Input: part model. Units: mm. Frame: model coordinates. A direction names the side the tool comes from. Round coordinates to 2 decimals unless told otherwise and drop trailing zeros. Loops run counter-clockwise (first coordinate to the right, second up) from the corner with the lowest first, then second, coordinate; pieces in that order, holes last. Notation, with made-up numbers: M 27.5,79 L 36.5,79 A25 cw 36.5,102 Z; hole C 47,-7.5 d6. An arc over 180 degrees is marked long. Return JSON: item names as keys, results as strings. Group by question number.
1) Section A-A (x = 47). Output: boundary loops of the cut face in (y, z).
2) Access query for faces 1 (the face through (67.71, -12.64, 2.81)), 2 (the face through (0, 0, 0)), 3 (the face through (137.62, -2.38, 10.74)), 4 (the face through (67, 12, 0)). Directions: +Z, -Z, +X, -X, +Y, -Y. A direction counts if a zero-diameter tool reaches every point of the face in a straight line with its end or side. Return the directions, or none.
3) Contact query for flat-ended pins moving along their axis: P1, Ø6, axis at x = 120.5, z = 9.5, coming from the +Y side; P2, Ø6, axis at y = -14, z = 11.5, coming from the -X side; P3, Ø8, axis at x = 48.5, z = -10, coming from the -Y side. Output: stop coordinate, or through.
4) Section B-B (z = -15.5). Output: boundary loops of the cut face in (x, y).
5) Mould query, pull axis Z, two halves, no side actions, for faces 5 (the face through (42, 12, 4)), 6 (the face through (90, 5, 10)), 7 (the face through (16.014, 8.767, 16.856)). Classes: +Z half, -Z half, draft (parallel to the pull), parting line (faces both ways), or undercut.
6) Material intervals for line 1 (X direction, y = 1.5, z = 13); line 2 (X direction, y = 13.5, z = 1.5); line 3 (X direction, y = 15, z = 2.5), sorted ascending. Write a range as from..to.
from build123d import *

# Parameters (mm, degrees)
CUT_EXTRUDE_START   = 10
CUT_EXTRUDE_1_DEPTH = 132.573302568
CUT_EXTRUDE_START_2 = 7
CUT_EXTRUDE_2_DEPTH = 135.573302568
CUT_EXTRUDE_START_3 = 68.5
SKETCH_4_R          = 14
SKETCH_4_R_2        = 12.95
CUT_EXTRUDE_3_DEPTH = 1.6
CUT_EXTRUDE_START_4 = 136.2
SKETCH_5_R          = 11
SKETCH_5_R_2        = 10.25
CUT_EXTRUDE_4_DEPTH = 1.3


with BuildPart() as part:
    # Эскиз1 → Повернуть1 (revolve)
    with BuildSketch(Plane.XY):
        Polygon((0, 0), (0, 12.5), (15, 12.5), (15, 14), (15, 19), (17, 19), (17, 14), (75, 14), (75, 12.5), (90, 12.5), (90, 11), (139, 11), (139, 0), align=None)
    revolve(axis=Axis((139, 0, 0), (-1, 0, 0)))

    # Эскиз2 → Вырез-Вытянуть1 (cut, through all)
    with BuildSketch(Plane(origin=(0, 0, 0), x_dir=(1, 0, 0), z_dir=(0, 1, 0)).offset(CUT_EXTRUDE_START)):
        with BuildLine():
            Line((21, 4), (63, 4))
            ThreePointArc((63, 4), (67, 0), (63, -4))
            Line((63, -4), (21, -4))
            ThreePointArc((21, -4), (17, 0), (21, 4))
        make_face()
    extrude(amount=CUT_EXTRUDE_1_DEPTH, mode=Mode.SUBTRACT)

    # Эскиз3 → Вырез-Вытянуть2 (cut, through all)
    with BuildSketch(Plane(origin=(0, 0, 0), x_dir=(1, 0, 0), z_dir=(0, 1, 0)).offset(CUT_EXTRUDE_START_2)):
        with BuildLine():
            Line((94, 4), (131, 4))
            ThreePointArc((131, 4), (135, 0), (131, -4))
            Line((131, -4), (94, -4))
            ThreePointArc((94, -4), (90, 0), (94, 4))
        make_face()
    extrude(amount=CUT_EXTRUDE_2_DEPTH, mode=Mode.SUBTRACT)

    # Эскиз4 → Вырез-Вытянуть3 (cut)
    with BuildSketch(Plane(origin=(0, 0, 0), x_dir=(0, 0, -1), z_dir=(1, 0, 0)).offset(CUT_EXTRUDE_START_3)):
        with Locations(Location((0, 0, 0), (0, 0, 90))):
            Circle(SKETCH_4_R)
        Circle(SKETCH_4_R_2, mode=Mode.SUBTRACT)
    extrude(amount=-CUT_EXTRUDE_3_DEPTH, mode=Mode.SUBTRACT)

    # Эскиз5 → Вырез-Вытянуть4 (cut)
    with BuildSketch(Plane(origin=(0, 0, 0), x_dir=(0, 0, -1), z_dir=(1, 0, 0)).offset(CUT_EXTRUDE_START_4)):
        with Locations(Location((0, 0, 0), (0, 0, 90))):
            Circle(SKETCH_5_R)
        Circle(SKETCH_5_R_2, mode=Mode.SUBTRACT)
    extrude(amount=-CUT_EXTRUDE_4_DEPTH, mode=Mode.SUBTRACT)


solid = part.part
Returned:
{
 "1": {"outline": "M 10,-4 L 10,4 L 13.42,4 A14 ccw long 13.42,-4 Z"},
 "2": {"face 1": "none", "face 2": "+Z, -Z, -X, +Y, -Y", "face 3": "+X", "face 4": "+Y"},
 "3": {"P1": "stops at y = 8.87", "P2": "stops at x = 15", "P3": "stops at y = -12.65"},
 "4": {"outline": "M 15,-10.99 L 17,-10.99 L 17,10.99 L 15,10.99 Z"},
 "5": {"face 5": "undercut", "face 6": "draft", "face 7": "parting line"},
 "6": {"line 1": "x = 15..66.9, 68.5..75", "line 2": "x = 15..17.29, 66.71..66.9, 68.5..75", "line 3": "x = 15..17"}
}
